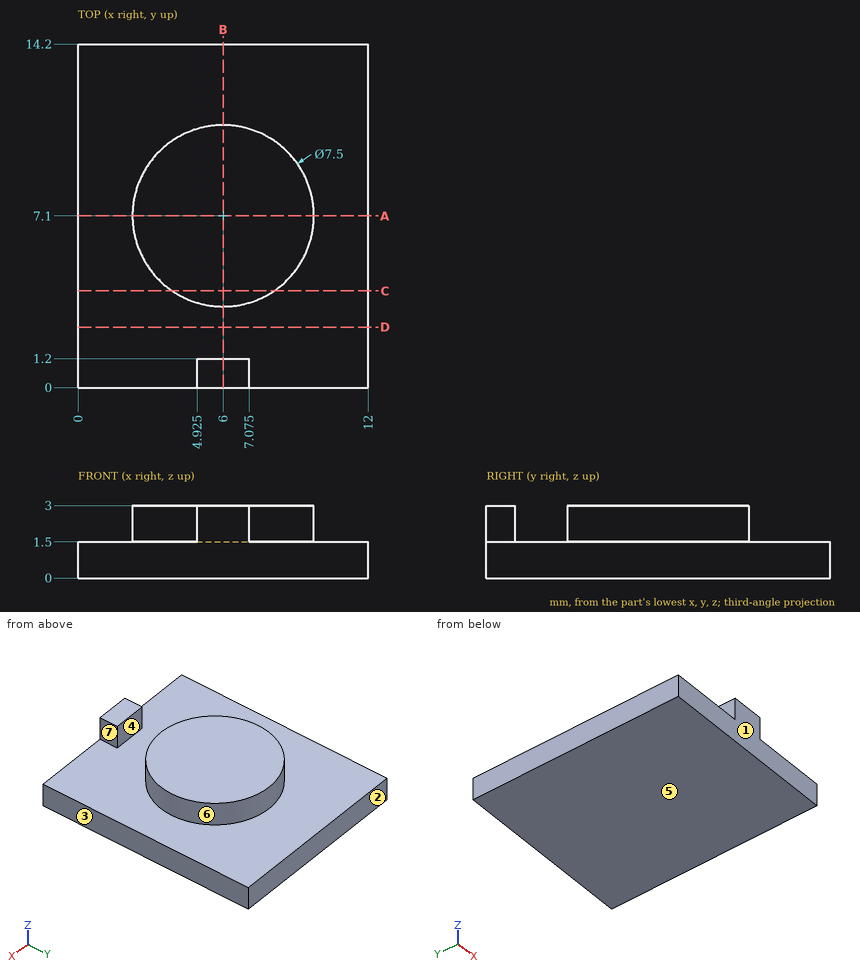
Here's the drawing with two shaded views (mm, measured from the low corner). I have some questions. A direction names the side the tool comes from. Give positions to 0.01 mm unless a question says otherwise; leave off trailing zeros. Loops run counter-clockwise (first coordinate to the right, second up) from the corner with the lowest first, then second, coordinate; pieces in that order, holes last. Notation, with made-up numbers: M -7.75,12 L 25.25,12 A10 cw 25.25,20 Z; hole C -11,84.5 d5. An arc over 180 degrees is marked long. One line per item, written item: value. Start each with the question number.
1) I'm going to push flat-ended pins straight in: pin 1 (0.6 mm diameter, centred on y = 0.5, z = 2, fed in from +X) (3 decimals); pin 2 (1.6 mm diameter, centred on x = 6, z = 2.5, fed in from +Y); pin 3 (1 mm diameter, centred on x = 6, y = 2, fed in from +Z). Where does each tip first touch, or does it pass through?
2) If we section it at B-B, the plane x = 6: Write out the boundary of the cut face in (y, z).
3) Thinking about a two-plate mould opening in Y: for the marked faces 1, 2, 3 and 4, which applies, +Y half, -Y half, draft (parallel to the pull), parting line (faces both ways), or undercut?
4) If we section it at C-C, the plane y = 4: Write out the boundary of the cut face in (x, z).
5) On a 3-axis mill with a long thin cutter (end or side, diameter ignored), from which of +Z, -Z, +X, -X, +Y, -Y can I reach the whole of each face in a straight line? I mean the marked faces 5, 6 and 7. Say none if no direction works.
6) If we section it at A-A, the plane y = 7.1: Write out the boundary of the cut face in (x, z).
7) If we section it at D-D, the plane y = 2.5: Write out the boundary of the cut face in (x, z), and give its area (3 significant figures).
8) If I drill on line 1 (Z direction, x = 0.5, y = 6); line 2 (Y direction, x = 8.75, z = 1.8); line 3 (X direction, y = 6, z = 1.8), over which ranges is the centre line in solid material (lowest first)? Write a range as [from, to].
Completed:
1. pin 1: stops at x = 7.075
1. pin 2: stops at y = 10.85
1. pin 3: stops at z = 1.5
2. outline: M 0,0 L 14.2,0 L 14.2,1.5 L 10.85,1.5 L 10.85,3 L 3.35,3 L 3.35,1.5 L 1.2,1.5 L 1.2,3 L 0,3 Z
3. face 1: -Y half
3. face 2: +Y half
3. face 3: draft
3. face 4: undercut
4. outline: M 0,0 L 12,0 L 12,1.5 L 8.11,1.5 L 8.11,3 L 3.89,3 L 3.89,1.5 L 0,1.5 Z
5. face 5: -Z, +X, -X, +Y, -Y
5. face 6: +Z
5. face 7: +Z, +X, -Y
6. outline: M 0,0 L 12,0 L 12,1.5 L 9.75,1.5 L 9.75,3 L 2.25,3 L 2.25,1.5 L 0,1.5 Z
7. outline: M 0,0 L 12,0 L 12,1.5 L 0,1.5 Z
7. area: 18.0 mm^2
8. line 1: z = [0, 1.5]
8. line 2: y = [4.55, 9.65]
8. line 3: x = [2.41, 9.59]
